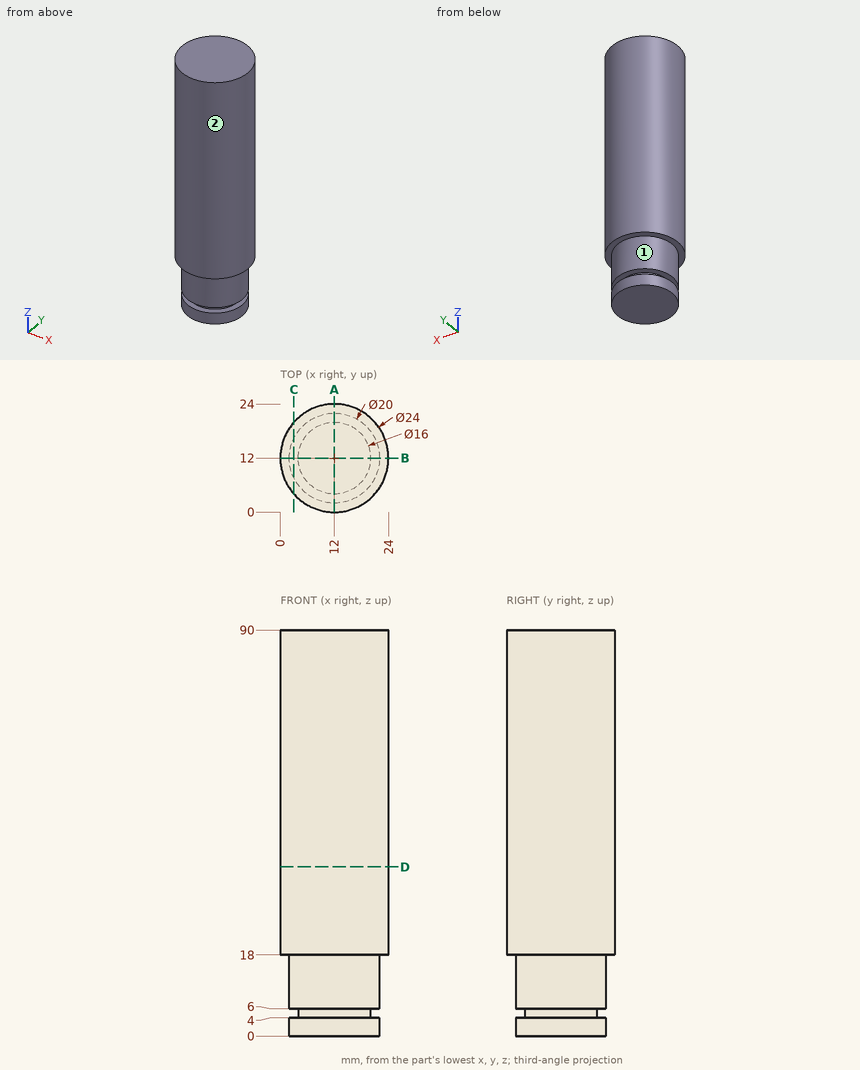
Input: dimensioned drawing with shaded views. Units: mm. Origin: part minimum x, y, z. A direction names the side the tool comes from. Round coordinates to 2 decimals unless told otherwise and drop trailing zeros. Order: outer loops, then holes, each group sorted by start corner. A loop starts at its lowest first (then second) coordinate and runs counter-clockwise, first axis right, second up.
1. Cut plane A-A, the plane x = 12. Output: boundary loops of the cut face in (y, z), then the cut area to 3 significant figures.
The answers:
outline: (0, 18) - (2, 18) - (2, 6) - (4, 6) - (4, 4) - (2, 4) - (2, 0) - (22, 0) - (22, 4) - (20, 4) - (20, 6) - (22, 6) - (22, 18) - (24, 18) - (24, 90) - (0, 90) - close
area: 2,080 mm2
2. Pin query (flat end, axial travel): P1, Ø3, axis at y = 13.5, z = 66, coming from the -X side; P2, Ø10, axis at x = 6.5, z = 76.5, coming from the -Y side; P3, Ø1.5, axis at x = 15, z = 12, coming from the +Y side; P4, Ø6, axis at x = 7, z = 46.5, coming from the +Y side. Return the tip coordinate at first contact, or that it passes through.
The answers:
P1: stops at x = 0
P2: stops at y = 0.01
P3: stops at y = 21.74
P4: stops at y = 23.83
3. Cut plane D-D, the plane z = 37.5. Output: boundary loops of the cut face in (x, y), then the cut area to 3 significant figures.
The answers:
outline: circle Ø24 at (12, 12)
area: 452 mm2
4. Set-up query: the marked faces 1 and 2. Return all of +Z, -Z, +X, -X, +Y, -Y with unobstructed straight access to the full face (end or side cutting, diameter ignored); none if empty.
The answers:
face 1: -Z
face 2: +Z, -Z
5. Material intervals for line 1 (X direction, y = 11.5, z = 64); line 2 (Z direction, x = 15.5, y = 1.5); line 3 (Z direction, x = 2.25, y = 11.25), sorted ascending.
The answers:
line 1: x = 0.01 to 23.99
line 2: z = 18 to 90
line 3: z = 0 to 4, 6 to 90
6. Cut plane C-C, the plane x = 3. Output: boundary loops of the cut face in (y, z), then the cut area to 3 significant figures.
The answers:
outline: (4.06, 18) - (7.64, 18) - (7.64, 6) - (16.36, 6) - (16.36, 18) - (19.94, 18) - (19.94, 90) - (4.06, 90) - close; (7.64, 0) - (16.36, 0) - (16.36, 4) - (7.64, 4) - close
area: 1,280 mm2
